from build123d import *

# Parameters (mm, degrees)
SKETCH1_W           = 3
SKETCH1_H           = 1
SKETCH1_W_2         = 1
SKETCH1_H_2         = 3
BOSS_EXTRUDE1_DEPTH = 15
SKETCH2_OUTSIDE_W   = 8.118
SKETCH2_OUTSIDE_H   = 8.118
SKETCH2_OUTSIDE_R   = 1.5
CUT_EXTRUDE1_DEPTH  = 15


with BuildPart() as part:
    # Sketch1 → Boss-Extrude1 (new body)
    with BuildSketch(Plane(origin=(0, 0, 0), x_dir=(1, 0, 0), z_dir=(0, 1, 0))):
        Rectangle(SKETCH1_W, SKETCH1_H)
        Rectangle(SKETCH1_W_2, SKETCH1_H_2)
    extrude(amount=BOSS_EXTRUDE1_DEPTH)

    # Sketch2 outside → Cut-Extrude1 (cut)
    with BuildSketch(Plane(origin=(0, 15, 0), x_dir=(1, 0, 0), z_dir=(0, 1, 0))):
        Rectangle(SKETCH2_OUTSIDE_W, SKETCH2_OUTSIDE_H)
        Circle(SKETCH2_OUTSIDE_R, mode=Mode.SUBTRACT)
    extrude(amount=-CUT_EXTRUDE1_DEPTH, mode=Mode.SUBTRACT)


solid = part.part
Here's how the part is built. I have some questions about the finished solid (model axes, mm). A direction names the side the tool comes from. Coordinates: 2 decimals unless noted, no trailing zeros. Loops run counter-clockwise (first coordinate to the right, second up) from the corner with the lowest first, then second, coordinate; pieces in that order, holes last.
1. For P1, Ø0.5, axis at y = 10.5, z = -1, coming from the +X side; P2, Ø0.7, axis at y = 11, z = 1, coming from the -X side; P3, Ø0.5, axis at x = 1, y = 7.5, coming from the -Z side, each with a flat end and sliding along its axis, tell me the tip position at first contact or that it passes through.
2. Imagine slicing it at B-B, the plane z = -0.8. Please give me the cut outline in (x, y).
3. For faces 4 (the flat face through (0.5, 7, 1)), 5 (the flat face through (-1, 7, 0.5)), 6 (the flat face through (-0.5, 7, -1)), which set-ups out of +Z, -Z, +X, -X, +Y, -Y let a thin tool reach every point of the face, with its end or its side?
4. I need wall thicknesses on L1, parallel to Z at x = -0.85, y = 7; L2, parallel to Z at x = -0.2, y = 5. Which ranges of each line are inside material? Lowest first, please.
5. Imagine slicing it at C-C, the plane x = 1.25. Please give me the cut outline in (y, z).
6. Imagine slicing it at A-A, the plane y = 9.75. Please give me the cut outline in (x, z), and give its area (3 significant figures).
7. If we mould it in two halves opening along Z, with no side actions, what happens to faces 1 (the flat face through (0, 15, 0)), 2 (the flat face through (1, 7, -0.5)), 3 (the flat face through (1, 7, 0.5))? For each: pulls with the +Z half, pulls with the -Z half, needs draft (parallel to the pull), parting line crosses it, or undercut.
Taken from the geometry:
1. P1: stops at x = 0.5
1. P2: stops at x = -0.5
1. P3: stops at z = -0.5
2. outline: (-0.5, 0) - (0.5, 0) - (0.5, 15) - (-0.5, 15) - close
3. face 4: +Z, +X, +Y, -Y
3. face 5: +Z, -X, +Y, -Y
3. face 6: -Z, -X, +Y, -Y
4. L1: z = -0.5 to 0.5
4. L2: z = -1.49 to 1.49
5. outline: (0, -0.5) - (15, -0.5) - (15, 0.5) - (0, 0.5) - close
6. outline: (-1.41, -0.5) - (-0.5, -0.5) - (-0.5, -1.41) arc R1.5 ccw to (0.5, -1.41) - (0.5, -0.5) - (1.41, -0.5) arc R1.5 ccw to (1.41, 0.5) - (0.5, 0.5) - (0.5, 1.41) arc R1.5 ccw to (-0.5, 1.41) - (-0.5, 0.5) - (-1.41, 0.5) arc R1.5 ccw to start
6. area: 4.89 mm2
7. face 1: needs draft
7. face 2: pulls with the -Z half
7. face 3: pulls with the +Z half
